Autodesk Inventor part; units mm, degrees
ref_plane "YZ Plane" through (0, 0, 0) normal (1, 0, 0) x (0, 1, 0)
ref_plane "XZ Plane" through (0, 0, 0) normal (0, 1, 0) x (-1, 0, 0)
ref_plane "XY Plane" through (0, 0, 0) normal (0, 0, 1) x (1, 0, 0)
sketch "Sketch1" plane through (0, 0, 0) normal (0, 0, 1) x (1, 0, 0)
  arc A0 (-38.9417, -24.6919) -> (-28.9986, -35.9017) centre (-34.2277, -30.5252) ccw
  arc A1 (40.4325, 20.1668) -> (31.0583, 31.8767) centre (35.7723, 26.0433) ccw
  arc A2 (-29.5767, 31.9271) -> (-38.9417, 20.21) centre (-34.2277, 26.0433) ccw
  arc A3 (31.0583, -36.3586) -> (40.1831, -24.4593) centre (35.7723, -30.5252) ccw
  line L0 (-16.5862, 21.6584) -> (18.4138, 21.6584)
  line L1 (-16.7484, -26.0092) -> (18.2516, -26.0092)
  line L2 (-20.4409, 5.259) -> (-20.4409, -9.741)
  line L3 (21.8055, 5.3953) -> (21.8055, -9.6047)
  circle A4 centre (-34.2277, 26.0433) radius 1.5
  circle A5 centre (35.7723, 26.0433) radius 1.5
  circle A6 centre (-34.2277, -30.5252) radius 1.5
  circle A7 centre (35.7723, -30.5252) radius 1.5
  circle A8 centre (-15.238, 13.5222) radius 1.5
  circle A9 centre (14.762, 13.5222) radius 1.5
  circle A10 centre (-15.238, -16.4778) radius 1.5
  circle A11 centre (14.762, -16.4778) radius 1.5
  line L4 (-34.2277, 26.0433) -> (-34.2277, 24.5433)
  line L5 (-34.2277, -29.0252) -> (-34.2277, -30.5252)
  line L6 (-38.9417, 20.21) -> (-20.4409, 5.259)
  line L7 (18.2516, -26.0092) -> (31.0583, -36.3586)
  line L8 (-15.238, 13.5222) -> (-15.238, 12.0222)
  line L9 (-15.238, -14.9778) -> (-15.238, -16.4778)
  line L10 (-38.9417, -24.6919) -> (-20.4409, -9.741)
  line L11 (35.7723, 26.0433) -> (35.7723, 24.5433)
  line L12 (34.2723, 26.0433) -> (35.7723, 26.0433)
  line L13 (40.7786, -24.9407) -> (21.8055, -9.6047)
  line L14 (-16.5862, 21.6584) -> (-29.5767, 31.9271)
  line L15 (-15.238, 15.0222) -> (-15.238, 13.5222)
  line L16 (18.4138, 21.6584) -> (31.0583, 31.8767)
  line L17 (-15.238, 13.5222) -> (-13.738, 13.5222)
  line L18 (13.262, 13.5222) -> (14.762, 13.5222)
  line L19 (14.762, 13.5222) -> (14.762, 12.0222)
  line L20 (14.762, -14.9778) -> (14.762, -16.4778)
  line L21 (14.762, -16.4778) -> (13.262, -16.4778)
  line L22 (-13.738, -16.4778) -> (-15.238, -16.4778)
  line L23 (-28.9986, -35.9017) -> (-16.7484, -26.0092)
  line L24 (21.8055, 5.3953) -> (40.4325, 20.1668)
  line L25 (35.7723, -30.5252) -> (34.2723, -30.5252)
  line L26 (-32.7277, -30.5252) -> (-34.2277, -30.5252)
  line L27 (35.7723, -29.0252) -> (35.7723, -30.5252)
  dimension "d27" = 3
  dimension "d6" = 15
  dimension "d7" = 15
  dimension "d9" = 15
  dimension "d10" = 15
  dimension "d16" = 90
  dimension "d17" = 90
  dimension "d20" = 70
  dimension "d23" = 35
  dimension "d24" = 35
  dimension "d25" = 15
  dimension "d26" = 15
  dimension "d28" = 3
  dimension "d29" = 3
  dimension "d30" = 3
  dimension "d33" = 30
  dimension "d35" = 30
  dimension "d37" = 30
  dimension "d39" = 3
  dimension "d40" = 3
  dimension "d41" = 3
  dimension "d42" = 3
  dimension "d45" = 70
  dimension "d46" = 56.5685
  dimension "d47" = 56.5685
extrude "Extrusion1" add sketch "Sketch1" along normal blind 2 contours L10 L2 L6 A2 L14 L0 L16 A1 L24 L3 L13 A3 L7 L1 L23 A0
sketch "Sketch2" plane through (0, 0, 2) normal (0, 0, 1) x (1, 0, 0)
  line L0 (-23.7277, 59.388) -> (25.2723, 59.388)
  line L1 (25.2723, -25.5399) -> (-23.7277, -25.5399)
  arc A0 (-23.7277, 59.388) -> (-27.2277, 55.888) centre (-23.7277, 55.888) ccw
  arc A1 (28.7723, 55.888) -> (25.2723, 59.388) centre (25.2723, 55.888) ccw
  arc A2 (-27.2277, -22.0399) -> (-23.7277, -25.5399) centre (-23.7277, -22.0399) ccw
  arc A3 (25.2723, -25.5399) -> (28.7723, -22.0399) centre (25.2723, -22.0399) ccw
  circle A4 centre (-23.7277, -22.0399) radius 1.375
  circle A5 centre (25.2723, -22.0399) radius 1.375
  circle A6 centre (-34.2277, -30.5252) radius 1.5
  circle A7 centre (-34.2277, 26.0433) radius 1.5
  circle A8 centre (35.7723, 26.0433) radius 1.5
  circle A9 centre (-15.238, -16.4778) radius 1.5
  circle A10 centre (14.762, -16.4778) radius 1.5
  circle A11 centre (14.762, 13.5222) radius 1.5
  circle A12 centre (35.7723, -30.5252) radius 1.5
  circle A13 centre (-34.2277, -30.5252) radius 1.5
  line L2 (40.7786, -24.9407) -> (21.8055, -9.6047)
  line L3 (21.8055, -9.6047) -> (21.8055, 5.3953)
  line L4 (21.8055, 5.3953) -> (40.4325, 20.1668)
  arc A14 (40.4325, 20.1668) -> (31.0583, 31.8767) centre (35.7723, 26.0433) ccw
  line L5 (31.0583, 31.8767) -> (18.4138, 21.6584)
  line L6 (18.4138, 21.6584) -> (-16.5862, 21.6584)
  line L7 (-16.5862, 21.6584) -> (-29.5767, 31.9271)
  arc A15 (-29.5767, 31.9271) -> (-38.9417, 20.21) centre (-34.2277, 26.0433) ccw
  line L8 (-38.9417, 20.21) -> (-20.4409, 5.259)
  line L9 (-20.4409, 5.259) -> (-20.4409, -9.741)
  line L10 (-20.4409, -9.741) -> (-38.9417, -24.6919)
  arc A16 (-38.9417, -24.6919) -> (-28.9986, -35.9017) centre (-34.2277, -30.5252) ccw
  line L11 (-28.9986, -35.9017) -> (-16.7484, -26.0092)
  line L12 (-16.7484, -26.0092) -> (18.2516, -26.0092)
  line L13 (18.2516, -26.0092) -> (31.0583, -36.3586)
  arc A17 (31.0583, -36.3586) -> (40.7786, -24.9407) centre (35.7723, -30.5252) ccw
  circle A18 centre (-15.238, 13.5222) radius 1.5
  circle A19 centre (35.7723, 26.0433) radius 1.5
  circle A20 centre (-34.2277, 26.0433) radius 1.5
  circle A21 centre (-23.7277, 35.9601) radius 1.375
  circle A22 centre (25.2723, 35.9601) radius 1.375
  line L14 (28.7723, 55.888) -> (28.7723, -22.0399)
  line L15 (28.7723, -24.8684) -> (28.7723, -25.5399)
  line L16 (-27.2277, -25.5399) -> (-27.2277, -24.8684)
  line L17 (-27.2277, -22.0399) -> (-27.2277, 55.888)
  line L18 (34.6056, 25.1005) -> (35.7723, 26.0433)
  line L19 (-34.2277, 26.0433) -> (-33.061, 25.1005)
  line L20 (-34.2277, -30.5252) -> (-33.061, -29.5824)
  line L21 (-27.2277, -24.8684) -> (-22.6582, -21.1757)
  line L22 (27.9945, -24.2398) -> (28.7723, -24.8684)
  line L23 (34.6056, -29.5824) -> (35.7723, -30.5252)
  point P0 (0, 0)
  dimension "d54" = 2.75
  dimension "d48" = 56
  dimension "d49" = 85
  dimension "d50" = 7
  dimension "d51" = 7
  dimension "d52" = 7
  dimension "d53" = 7
  dimension "d55" = 2.75
  dimension "d56" = 2.75
  dimension "d57" = 2.75
  dimension "d58" = 58
  dimension "d59" = 58
extrude "Extrusion2" add sketch "Sketch2" along normal blind 2 contours L0 A1 L14 L5 L6 L7 L17 A0 | L7 L6 L5 L14 L4 L3 L2 A3 L1 A2 L17 L10 L9 L8 | L8 L9 L10 L17 | L14 L2 L3 L4
hole "Hole1" at (-23.7277, -22.0399, 4) direction (0, 0, -1) diameter 3 end through all
hole "Hole2" at (25.2723, -22.0399, 2) direction (0, 0, -1) diameter 3 end through all
equation "\"d24\" = d23"
properties part number "ChasisInferiorDron_P9"
The model under review builds one solid part; all positions refer to its coordinate system, in mm. A direction names the side the tool comes from. Coordinates: 2 decimals unless noted, no trailing zeros. Loops run counter-clockwise (first coordinate to the right, second up) from the corner with the lowest first, then second, coordinate; pieces in that order, holes last. Notation, with made-up numbers: M 5,38.5 L 36,38.5 A12 ccw 36,46.5 Z; hole C -30.75,70 d4. An arc over 180 degrees is marked long. Put each result on its own line as item: value. Start each with the question number.
Q1. For faces 4 (the flat face through (24.565, -31.111, 0.986)), 5 (the flat face through (34, 25, 2)), 6 (the cylindrical face through (27.77, -24.49, 2.99)), 7 (the flat face through (-27.228, 16, 3)), 8 (the flat face through (24.65, 26.7, 0.99)), list the 3-axis set-ups (+Z, -Z, +X, -X, +Y, -Y) from which the entire face can be reached by the end or side of a thin tool; tool diameter is ignored.
Q2. Clearance check with flat-ended pins moving along their axes: pin 1 (1 mm diameter, centred on x = -8, z = 0.5, fed in from -Y); pin 2 (16 mm diameter, centred on x = -36.5, y = 21.5, fed in from +Z); pin 3 (2 mm diameter, centred on y = -5, z = 0.5, fed in from -X). State where each tip first meets the part, or that it passes through.
Q3. Add section A-A (x = 3). Write out the cut boundary in (y, z), and give its area (3 significant figures).
Q4. The part is to be moulded in two halves that separate along Y. For faces 1 (the cylindrical face through (-22.416, 35.547, 2.986)), 2 (the flat face through (1, 21.658, 1)), 3 (the flat face through (28.772, 17, 3)), say which applies: +Y half, -Y half, draft (parallel to the pull), parting line (faces both ways), or undercut.
Q5. Add section D-D (y = 51). Write out the cut boundary in (x, z).
Q6. Add section C-C (z = 0.85). Count the separate pieces of the cut face and the enclosed holes in it, and give its area (3 significant figures).
Q7. Add section B-B (y = -7.5). Write out the cut boundary in (x, z).
Q8. Wall thickness on line 1 (Y direction, x = -25, z = 0.8); line 2 (Y direction, x = 26.5, z = 2.45); line 3 (X direction, y = 12.5, z = 2.3): over which ranges is each line inside the solid? List them lowest first.
Answers:
1. face 4: +Z, -Z, -Y
1. face 5: +Z, +X, +Y, -Y
1. face 6: +Z, +X, -Y
1. face 7: +Z, -X, +Y, -Y
1. face 8: -Z, +Y
2. pin 1: stops at y = -26.01
2. pin 2: stops at z = 2
2. pin 3: stops at x = -20.44
3. outline: M -26.01,0 L 21.66,0 L 21.66,2 L 59.39,2 L 59.39,4 L -25.54,4 L -25.54,2 L -26.01,2 Z
3. area: 265 mm^2
4. face 1: undercut
4. face 2: +Y half
4. face 3: draft
5. outline: M -27.23,2 L 28.77,2 L 28.77,4 L -27.23,4 Z
6. separate pieces: 1
6. enclosed holes: 10
6. area: 3,390 mm^2
7. outline: M -27.23,2 L -20.44,2 L -20.44,0 L 21.81,0 L 21.81,2 L 28.77,2 L 28.77,4 L -27.23,4 Z
8. line 1: y = -32.67 to -22.83, -21.25 to -13.43, 8.94 to 28.31
8. line 2: y = -25.32 to -22.66, -21.42 to 35.34, 36.58 to 59.17
8. line 3: x = -27.23 to -16.34, -14.14 to 13.66, 15.86 to 28.77
